Here's how the part is built. I have some questions about the finished solid (model axes, mm). A direction names the side the tool comes from. Give positions to 0.01 mm unless a question says otherwise; leave off trailing zeros. Loops run counter-clockwise (first coordinate to the right, second up) from the corner with the lowest first, then second, coordinate; pieces in that order, holes last. Notation, with made-up numbers: (65, -34.5) - (86, -34.5) arc R23 cw to (86, -8.5) - close; hole circle Ø2 at (-11.75, -37). An arc over 180 degrees is marked (long way). Use one line per item in the form item = value.
from build123d import *

# Parameters (mm, degrees)
F0_W     = 5.501232
F0_H     = 10.183676
F1_DEPTH = 6.35


with BuildPart() as f1:
    # F0 (on Top) → F1 (new body)
    with BuildSketch(Plane.XY):
        with BuildLine():
            Line((-21.024568, 0), (-23.102842, 0))
            Line((-23.102842, 0), (-23.102842, -5.053747))
            Line((-23.102842, -5.053747), (-8.269768, -5.053747))
            ThreePointArc((-8.269768, -5.053747), (1.247028, -12.800027), (10.763824, -5.053747))
            Line((10.763824, -5.053747), (10.763824, -2.526873))
            ThreePointArc((10.763824, -2.526873), (19.230491, -5.20295), (27.697158, -2.526873))
            Line((27.697158, -2.526873), (27.697158, 15.555039))
            Line((27.697158, 15.555039), (27.697158, 20.280621))
            Line((27.697158, 20.280621), (10.763824, 20.280621))
            Line((10.763824, 20.280621), (10.763824, 23.563793))
            ThreePointArc((10.763824, 23.563793), (7.258244, 27.516062), (2.289737, 29.311463))
            ThreePointArc((2.289737, 29.311463), (1.14428, 29.361855), (0, 29.289493))
            ThreePointArc((0, 29.289493), (-4.848945, 27.457979), (-8.269768, 23.563793))
            Line((-8.269768, 23.563793), (-8.269768, 13.323515))
            Line((-8.269768, 13.323515), (-10.668843, 16.080103))
            Line((-10.668843, 16.080103), (-15.686305, 16.080103))
            Line((-15.686305, 16.080103), (-20.0435, 16.080103))
            Line((-20.0435, 16.080103), (-21.024568, 16.080103))
            ThreePointArc((-21.024568, 16.080103), (-22.508695, 15.456849), (-23.102842, 13.960832))
            Line((-23.102842, 13.960832), (-23.102842, 12.142118))
            Line((-23.102842, 12.142118), (-23.102842, 8.040052))
            Line((-23.102842, 8.040052), (-23.102842, 2.839885))
            Line((-23.102842, 2.839885), (-21.024568, 0))
        make_face()
        with Locations((-15.551776, 7.931723)):
            Rectangle(F0_W, F0_H, mode=Mode.SUBTRACT)
        with BuildLine():
            Line((0, -5.053747), (0, 0))
            Line((0, 0), (-8.269768, 0))
            Line((-8.269768, 0), (-10.123806, 0))
            ThreePointArc((-10.123806, 0), (-8.76723, 1.336218), (-8.269768, 3.174236))
            Line((-8.269768, 3.174236), (-8.269768, 12.50577))
            Line((-8.269768, 12.50577), (4.200517, -0.817745))
            Line((4.200517, -0.817745), (4.200517, -5.053747))
            Line((4.200517, -5.053747), (0, -5.053747))
        make_face(mode=Mode.SUBTRACT)
        with BuildLine():
            Line((15.620673, 15.555039), (23.102842, 15.555039))
            Line((23.102842, 15.555039), (23.102842, 0))
            ThreePointArc((23.102842, 0), (19.361757, -1.116151), (15.620673, 0))
            Line((15.620673, 0), (15.620673, 15.555039))
        make_face(mode=Mode.SUBTRACT)
        Polygon((10.763824, 15.555039), (10.763824, 0), (-2.362791, 16.080103), (-2.362791, 20.280621), (4.988113, 20.280621), (4.988113, 15.555039), align=None, mode=Mode.SUBTRACT)
    extrude(amount=F1_DEPTH)


solid = f1.part
(1) For P1, Ø1.5, axis at x = 15.5, z = 4.5, coming from the +Y side; P2, Ø1, axis at y = 22.5, z = 4.5, coming from the +X side; P3, Ø3, axis at x = -16, z = 2, coming from the -Y side, each with a flat end and sliding along its axis, tell me the tip position at first contact or that it passes through.
Geometry says:
P1 = 20.28
P2 = 10.76
P3 = -5.05
(2) Thinking about a two-plate mould opening in X: for faces 4 (the flat face through (-23.103, 8, 3)), 5 (the flat face through (2, 9, 6.35)), 6 (the flat face through (-5, 0, 3)), which applies, pulls with the +X half, pulls with the -X half, needs draft (parallel to the pull), parting line crosses it, or undercut?
Geometry says:
face_4 = pulls with the -X half
face_5 = needs draft
face_6 = undercut
(3) If I drill on probe 1 along X at (y, z) = (16.5, 2.25); probe 2 along Y at (x, z) = (-13, 1.5); probe 3 along X at (y, z) = (-4, 3.5), over which ranges is the centre line in solid material (lowest first)?
Geometry says:
probe_1 = -8.27 to -2.36, 4.99 to 27.7
probe_2 = -5.05 to 2.84, 13.02 to 16.08
probe_3 = -23.1 to 0, 4.2 to 10.76, 13.4 to 25.06
(4) If we section it at C-C (y = 11): List the corners of the cut face in (x, z) for me.
Geometry says:
outline = (-23.1, 0) - (-18.3, 0) - (-18.3, 6.35) - (-23.1, 6.35) - close; (-12.8, 0) - (-8.27, 0) - (-8.27, 6.35) - (-12.8, 6.35) - close; (-6.86, 0) - (1.78, 0) - (1.78, 6.35) - (-6.86, 6.35) - close; (10.76, 0) - (15.62, 0) - (15.62, 6.35) - (10.76, 6.35) - close; (23.1, 0) - (27.7, 0) - (27.7, 6.35) - (23.1, 6.35) - close
(5) If we section it at D-D (z = 2.25): Give the number of separate pieces and of enclosed holes in the cut face, plus the area to 3 significant figures.
Geometry says:
separate_pieces = 1
enclosed_holes = 4
area = 1,050 mm²
(6) If we section it at B-B (x = -17): List the corners of the cut face in (y, z) for me.
Geometry says:
outline = (-5.05, 0) - (2.84, 0) - (2.84, 6.35) - (-5.05, 6.35) - close; (13.02, 0) - (16.08, 0) - (16.08, 6.35) - (13.02, 6.35) - close
(7) If we section it at A-A (y = 18): List the corners of the cut face in (x, z) for me, plus the area to 3 significant figures.
Geometry says:
outline = (-8.27, 0) - (-2.36, 0) - (-2.36, 6.35) - (-8.27, 6.35) - close; (4.99, 0) - (27.7, 0) - (27.7, 6.35) - (4.99, 6.35) - close
area = 182 mm²
(8) For faces 1 (the flat face through (-18.302, 8, 3)), 2 (the flat face through (-8.27, 19, 3)), 3 (the flat face through (-16, -5.054, 3)), which set-ups out of +Z, -Z, +X, -X, +Y, -Y let a thin tool reach every point of the face, with its end or its side?
Geometry says:
face_1 = +Z, -Z
face_2 = +Z, -Z, +Y
face_3 = +Z, -Z, -X, -Y
